For this review, take the finished solid that the model builds, in its own axes (mm). A direction names the side the tool comes from. Give positions to 0.01 mm unless a question says otherwise; leave off trailing zeros. Write each loop counter-clockwise with the first axis right and the second up, starting at its lowest first coordinate (ties: lowest second). Pieces come first, ordered by that corner, then holes.
Q1. Insertion check: P1, Ø12.5, axis at y = 8, z = 60.5, coming from the +X side; P2, Ø9, axis at x = 42.5, y = -6.5, coming from the +Z side; P3, Ø9, axis at x = 6.5, y = -24.5, coming from the +Z side. Each pin has a flat end and moves straight along its axis. Give the tip position at first contact, or say it passes through.
Q2. We need section B-B (z = 73). Write out the cut boundary in (x, y), then the cut area to 3 significant figures.
Q3. For line 1 (Y direction, x = 40, z = 16); line 2 (Z direction, x = 0, y = 12); line 3 (Z direction, x = 2.5, y = -13), list the stretches that pass through material, from the lowest coordinate up.
Q4. Mouldability with a two-part tool opening along Y and no side actions: class faces 5 (the flat face through (44, 20, 41)), 6 (the cylindrical face through (38.698, -10.085, 12.675)), 7 (the flat face through (-1, 0, 0)), 8 (the flat face through (-1, 35, 44)) as released by +Y, released by -Y, zero draft, split by the parting line, or undercut.
Q5. We need section C-C (y = 25.5). Write out the cut boundary in (x, z), then the cut area to 3 significant figures.
Q6. We need section A-A (x = 0). Write out the cut boundary in (y, z), then the cut area to 3 significant figures.
Q7. Machinability: for faces 1 (the flat face through (-44, 20, 41)), 2 (the flat face through (-35, 15, 80)), 3 (the flat face through (0, -20, 13)), 4 (the flat face through (35, 15, 80)), which of the approach directions +Z, -Z, +X, -X, +Y, -Y give a long, thin tool a straight path to every point of the face, cutting with its end or side? Answer none if there is none.
Q8. We need section D-D (z = 7). Write out the cut boundary in (x, y), then the cut area to 3 significant figures.
```python
from build123d import *

# Parameters (mm, degrees)
SKETCH_W        = 110
SKETCH_H        = 70
PAD_DEPTH       = 25
SKETCH001_W     = 50
SKETCH001_H     = 12
POCKET_DEPTH    = 70.001
PAD001_DEPTH    = 40
SKETCH003_R     = 16
POCKET001_DEPTH = 70.001
SKETCH004_W     = 15
SKETCH004_H     = 55
POCKET002_DEPTH = 25
POCKET003_DEPTH = 15.001
FILLET_R        = 6
FILLET001_R     = 6
FILLET002_R     = 16
SKETCH006_R     = 10
POCKET004_DEPTH = 25.001


with BuildPart() as part:
    # Sketch → Pad (new body)
    with BuildSketch(Plane.XY):
        Rectangle(SKETCH_W, SKETCH_H)
    extrude(amount=PAD_DEPTH)

    # Sketch001 (on Face3 of Pad) → Pocket (cut, through all)
    with BuildSketch(Plane.XZ.offset(35)):
        with Locations((0, 19)):
            Rectangle(SKETCH001_W, SKETCH001_H)
    extrude(amount=-POCKET_DEPTH, mode=Mode.SUBTRACT)

    # Sketch002 (on Face1 of Pocket) → Pad001 (join)
    with BuildSketch(Plane(origin=(0, 35, 0), x_dir=(-1, 0, 0), z_dir=(0, 1, 0))):
        with BuildLine():
            Line((-55, 25), (-55, 80))
            Line((-55, 80), (-30, 80))
            ThreePointArc((30, 80), (0, 110), (-30, 80))
            Line((55, 80), (30, 80))
            Line((55, 25), (55, 80))
            Line((25, 25), (55, 25))
            Line((25, 13), (25, 25))
            Line((-25, 13), (25, 13))
            Line((-25, 25), (-25, 13))
            Line((-55, 25), (-25, 25))
        make_face()
    extrude(amount=-PAD001_DEPTH)

    # Sketch003 (on Face4 of Pad001) → Pocket001 (cut, through all)
    with BuildSketch(Plane(origin=(0, 35, 0), x_dir=(-1, 0, 0), z_dir=(0, 1, 0))):
        with Locations((0, 80)):
            Circle(SKETCH003_R)
    extrude(amount=-POCKET001_DEPTH, mode=Mode.SUBTRACT)

    # Sketch004 (on Face18 of Pocket001) → Pocket002 (cut)
    with BuildSketch(Plane.XZ.offset(5)):
        with Locations((-47.5, 52.5)):
            Rectangle(SKETCH004_W, SKETCH004_H)
        with Locations((47.5, 52.5)):
            Rectangle(SKETCH004_W, SKETCH004_H)
    extrude(amount=-POCKET002_DEPTH, mode=Mode.SUBTRACT)

    # Sketch005 (on Face24 of Pocket002) → Pocket003 (cut, through all)
    with BuildSketch(Plane.XZ.offset(-20)):
        Polygon((-55, 80), (-55, 25), (-40, 80), align=None)
        Polygon((55, 25), (40, 80), (55, 80), align=None)
    extrude(amount=-POCKET003_DEPTH, mode=Mode.SUBTRACT)

    # Fillet
    fillet_edges = [part.edges().sort_by_distance(p)[0] for p in [
        (25, -20, 13),
    ]]
    fillet(fillet_edges, radius=FILLET_R)

    # Fillet001
    fillet001_edges = [part.edges().sort_by_distance(p)[0] for p in [
        (-25, -20, 13),
    ]]
    fillet(fillet001_edges, radius=FILLET001_R)

    # Fillet002
    fillet002_edges = [part.edges().sort_by_distance(p)[0] for p in [
        (-55, -35, 12.5),
        (55, -35, 12.5),
    ]]
    fillet(fillet002_edges, radius=FILLET002_R)

    # Sketch006 (on Face2 of Fillet002) → Pocket004 (cut, through all)
    with BuildSketch(Plane.XY.offset(25)):
        with Locations((-40, -20)):
            Circle(SKETCH006_R)
        with Locations((40, -20)):
            Circle(SKETCH006_R)
    extrude(amount=-POCKET004_DEPTH, mode=Mode.SUBTRACT)


solid = part.part
```
Computed:
1. P1: stops at x = 40
1. P2: stops at z = 80
1. P3: stops at z = 13
2. outline: (-41.91, 20) - (-40, 20) - (-40, -5) - (-14.39, -5) - (-14.39, 35) - (-41.91, 35) - close; (14.39, -5) - (40, -5) - (40, 20) - (41.91, 20) - (41.91, 35) - (14.39, 35) - close
2. area: 2,110 mm2
3. line 1: y = -34.97 to -30, -10 to 35
3. line 2: z = 0 to 64, 96 to 110
3. line 3: z = 0 to 13
4. face 5: released by -Y
4. face 6: undercut
4. face 7: zero draft
4. face 8: released by +Y
5. outline: (-55, 0) - (55, 0) - (55, 25) - (40, 80) - (30, 80) arc R30 ccw to (-30, 80) - (-40, 80) - (-55, 25) - close; hole circle Ø32 at (0, 80)
5. area: 8,580 mm2
6. outline: (-35, 0) - (35, 0) - (35, 64) - (-5, 64) - (-5, 13) - (-35, 13) - close; (-5, 96) - (35, 96) - (35, 110) - (-5, 110) - close
6. area: 3,510 mm2
7. face 1: +Z, -X, -Y
7. face 2: +Z, -X, +Y, -Y
7. face 3: +Z, -Y
7. face 4: +Z, +X, +Y, -Y
8. outline: (-55, -19) arc R16 ccw to (-39, -35) - (39, -35) arc R16 ccw to (55, -19) - (55, 35) - (-55, 35) - close; hole circle Ø20 at (-40, -20); hole circle Ø20 at (40, -20)
8. area: 6,960 mm2
